The listing builds one solid part. Answer for the finished solid, in the listing's coordinates (mm). A direction names the side the tool comes from. Give positions to 0.01 mm unless a question says otherwise; leave off trailing zeros. Write each question's results on one line, items separated by ' | '. Start each with the question number.
from build123d import *

# Parameters (mm, degrees)
SKETCH1_W           = 38.1
SKETCH1_H           = 19.05
SKETCH1_W_2         = 31.75
SKETCH1_H_2         = 12.7
BOSS_EXTRUDE1_DEPTH = 304.8
SKETCH2_R           = 14.2875
CUT_EXTRUDE1_DEPTH  = 20.05
SKETCH3_R           = 3.175
CUT_EXTRUDE2_DEPTH  = 20.05
CUT_EXTRUDE3_DEPTH  = 20.05
CUT_EXTRUDE6_DEPTH  = 39.1
CUT_EXTRUDE7_REACH  = 21.05
CUT_EXTRUDE8_REACH  = 21.05
SKETCH9_R           = 6.35
CUT_EXTRUDE9_REACH  = 21.05
SKETCH10_R          = 2.667
SKETCH11_R          = 6.35
CUT_EXTRUDE10_DEPTH = 20.05
CUT_EXTRUDE11_DEPTH = 20.05


with BuildPart() as part:
    # Sketch1 → Boss-Extrude1 (new body)
    with BuildSketch(Plane.XY):
        with Locations((19.05, 9.525)):
            Rectangle(SKETCH1_W, SKETCH1_H)
        with Locations((19.05, 9.525)):
            Rectangle(SKETCH1_W_2, SKETCH1_H_2, mode=Mode.SUBTRACT)
    extrude(amount=BOSS_EXTRUDE1_DEPTH)

    # Sketch2 → Cut-Extrude1 (cut, through all)
    with BuildSketch(Plane(origin=(0, 19.05, 0), x_dir=(1, 0, 0), z_dir=(0, 1, 0))):
        with Locations((19.05, -19.05)):
            Circle(SKETCH2_R)
        with Locations((19.05, -222.25)):
            Circle(SKETCH2_R)
    extrude(amount=-CUT_EXTRUDE1_DEPTH, mode=Mode.SUBTRACT)

    # Sketch3 → Cut-Extrude2 (cut, through all)
    with BuildSketch(Plane(origin=(0, 19.05, 0), x_dir=(1, 0, 0), z_dir=(0, 1, 0))):
        with Locations((19.05, -295.275)):
            Circle(SKETCH3_R)
    extrude(amount=-CUT_EXTRUDE2_DEPTH, mode=Mode.SUBTRACT)

    # Sketch4 → Cut-Extrude3 (cut, through all)
    with BuildSketch(Plane(origin=(0, 19.05, 0), x_dir=(1, 0, 0), z_dir=(0, 1, 0))):
        with BuildLine():
            Line((31.75, -304.8), (31.75, -247.65))
            ThreePointArc((31.75, -247.65), (33.609871939, -243.159871939), (38.1, -241.3))
            Line((38.1, -241.3), (38.1, -304.8))
            Line((38.1, -304.8), (31.75, -304.8))
        make_face()
    extrude(amount=-CUT_EXTRUDE3_DEPTH, mode=Mode.SUBTRACT)

    # Sketch7 → Cut-Extrude6 (cut, through all)
    with BuildSketch(Plane.ZY):
        with BuildLine():
            Line((19.05, 14.2875), (57.15, 14.2875))
            ThreePointArc((57.15, 14.2875), (61.9125, 9.525), (57.15, 4.7625))
            Line((57.15, 4.7625), (19.05, 4.7625))
            ThreePointArc((19.05, 4.7625), (14.2875, 9.525), (19.05, 14.2875))
        make_face()
        with BuildLine():
            Line((76.2, 14.2875), (114.3, 14.2875))
            ThreePointArc((114.3, 14.2875), (119.0625, 9.525), (114.3, 4.7625))
            Line((114.3, 4.7625), (76.2, 4.7625))
            ThreePointArc((76.2, 4.7625), (71.4375, 9.525), (76.2, 14.2875))
        make_face()
        with BuildLine():
            Line((133.35, 14.2875), (171.45, 14.2875))
            ThreePointArc((171.45, 14.2875), (176.2125, 9.525), (171.45, 4.7625))
            Line((171.45, 4.7625), (133.35, 4.7625))
            ThreePointArc((133.35, 4.7625), (128.5875, 9.525), (133.35, 14.2875))
        make_face()
        with BuildLine():
            Line((190.5, 14.2875), (228.6, 14.2875))
            ThreePointArc((228.6, 14.2875), (233.3625, 9.525), (228.6, 4.7625))
            Line((228.6, 4.7625), (190.5, 4.7625))
            ThreePointArc((190.5, 4.7625), (185.7375, 9.525), (190.5, 14.2875))
        make_face()
        with BuildLine():
            Line((247.65, 14.2875), (285.75, 14.2875))
            ThreePointArc((285.75, 14.2875), (290.5125, 9.525), (285.75, 4.7625))
            Line((285.75, 4.7625), (247.65, 4.7625))
            ThreePointArc((247.65, 4.7625), (242.8875, 9.525), (247.65, 14.2875))
        make_face()
    extrude(amount=-CUT_EXTRUDE6_DEPTH, mode=Mode.SUBTRACT)

    # Sketch8 → Cut-Extrude7 (cut, up to next)
    with BuildSketch(Plane(origin=(0, 19.05, 0), x_dir=(1, 0, 0), z_dir=(0, 1, 0)), mode=Mode.PRIVATE) as cut_extrude7_sk1:
        with BuildLine():
            Line((11.1125, -44.45), (26.9875, -44.45))
            ThreePointArc((26.9875, -44.45), (31.477628061, -46.309871939), (33.3375, -50.8))
            Line((33.3375, -50.8), (33.3375, -190.5))
            ThreePointArc((33.3375, -190.5), (31.477628061, -194.990128061), (26.9875, -196.85))
            Line((26.9875, -196.85), (11.1125, -196.85))
            ThreePointArc((11.1125, -196.85), (6.622371939, -194.990128061), (4.7625, -190.5))
            Line((4.7625, -190.5), (4.7625, -50.8))
            ThreePointArc((4.7625, -50.8), (6.622371939, -46.309871939), (11.1125, -44.45))
        make_face()
    cut_extrude7_tool1 = extrude(cut_extrude7_sk1.sketch, amount=-CUT_EXTRUDE7_REACH, mode=Mode.PRIVATE) & part.part
    add(cut_extrude7_tool1.solids().sort_by_distance((19.05, 19.05, 120.65))[0], mode=Mode.SUBTRACT)

    # Sketch9 → Cut-Extrude8 (cut, up to next)
    with BuildSketch(Plane.XZ, mode=Mode.PRIVATE) as cut_extrude8_sk1:
        with Locations((9.525, 48.475738686)):
            Circle(SKETCH9_R)
    cut_extrude8_tool1 = extrude(cut_extrude8_sk1.sketch, amount=-CUT_EXTRUDE8_REACH, mode=Mode.PRIVATE) & part.part
    add(cut_extrude8_tool1.solids().sort_by_distance((9.525, 0, 48.475739))[0], mode=Mode.SUBTRACT)
    # Sketch9 → Cut-Extrude8 (cut, up to next)
    with BuildSketch(Plane.XZ, mode=Mode.PRIVATE) as cut_extrude8_sk2:
        with Locations((28.575, 59.474261314)):
            Circle(SKETCH9_R)
    cut_extrude8_tool2 = extrude(cut_extrude8_sk2.sketch, amount=-CUT_EXTRUDE8_REACH, mode=Mode.PRIVATE) & part.part
    add(cut_extrude8_tool2.solids().sort_by_distance((28.575, 0, 59.474261))[0], mode=Mode.SUBTRACT)
    # Sketch9 → Cut-Extrude8 (cut, up to next)
    with BuildSketch(Plane.XZ, mode=Mode.PRIVATE) as cut_extrude8_sk3:
        with Locations((9.525, 67.525738686)):
            Circle(SKETCH9_R)
    cut_extrude8_tool3 = extrude(cut_extrude8_sk3.sketch, amount=-CUT_EXTRUDE8_REACH, mode=Mode.PRIVATE) & part.part
    add(cut_extrude8_tool3.solids().sort_by_distance((9.525, 0, 67.525739))[0], mode=Mode.SUBTRACT)
    # Sketch9 → Cut-Extrude8 (cut, up to next)
    with BuildSketch(Plane.XZ, mode=Mode.PRIVATE) as cut_extrude8_sk4:
        with Locations((28.575, 78.524261314)):
            Circle(SKETCH9_R)
    cut_extrude8_tool4 = extrude(cut_extrude8_sk4.sketch, amount=-CUT_EXTRUDE8_REACH, mode=Mode.PRIVATE) & part.part
    add(cut_extrude8_tool4.solids().sort_by_distance((28.575, 0, 78.524261))[0], mode=Mode.SUBTRACT)
    # Sketch9 → Cut-Extrude8 (cut, up to next)
    with BuildSketch(Plane.XZ, mode=Mode.PRIVATE) as cut_extrude8_sk5:
        with Locations((9.525, 86.575738686)):
            Circle(SKETCH9_R)
    cut_extrude8_tool5 = extrude(cut_extrude8_sk5.sketch, amount=-CUT_EXTRUDE8_REACH, mode=Mode.PRIVATE) & part.part
    add(cut_extrude8_tool5.solids().sort_by_distance((9.525, 0, 86.575739))[0], mode=Mode.SUBTRACT)
    # Sketch9 → Cut-Extrude8 (cut, up to next)
    with BuildSketch(Plane.XZ, mode=Mode.PRIVATE) as cut_extrude8_sk6:
        with Locations((28.575, 97.574261314)):
            Circle(SKETCH9_R)
    cut_extrude8_tool6 = extrude(cut_extrude8_sk6.sketch, amount=-CUT_EXTRUDE8_REACH, mode=Mode.PRIVATE) & part.part
    add(cut_extrude8_tool6.solids().sort_by_distance((28.575, 0, 97.574261))[0], mode=Mode.SUBTRACT)
    # Sketch9 → Cut-Extrude8 (cut, up to next)
    with BuildSketch(Plane.XZ, mode=Mode.PRIVATE) as cut_extrude8_sk7:
        with Locations((9.525, 105.625738686)):
            Circle(SKETCH9_R)
    cut_extrude8_tool7 = extrude(cut_extrude8_sk7.sketch, amount=-CUT_EXTRUDE8_REACH, mode=Mode.PRIVATE) & part.part
    add(cut_extrude8_tool7.solids().sort_by_distance((9.525, 0, 105.625739))[0], mode=Mode.SUBTRACT)
    # Sketch9 → Cut-Extrude8 (cut, up to next)
    with BuildSketch(Plane.XZ, mode=Mode.PRIVATE) as cut_extrude8_sk8:
        with Locations((28.575, 116.624261314)):
            Circle(SKETCH9_R)
    cut_extrude8_tool8 = extrude(cut_extrude8_sk8.sketch, amount=-CUT_EXTRUDE8_REACH, mode=Mode.PRIVATE) & part.part
    add(cut_extrude8_tool8.solids().sort_by_distance((28.575, 0, 116.624261))[0], mode=Mode.SUBTRACT)
    # Sketch9 → Cut-Extrude8 (cut, up to next)
    with BuildSketch(Plane.XZ, mode=Mode.PRIVATE) as cut_extrude8_sk9:
        with Locations((9.525, 124.675738686)):
            Circle(SKETCH9_R)
    cut_extrude8_tool9 = extrude(cut_extrude8_sk9.sketch, amount=-CUT_EXTRUDE8_REACH, mode=Mode.PRIVATE) & part.part
    add(cut_extrude8_tool9.solids().sort_by_distance((9.525, 0, 124.675739))[0], mode=Mode.SUBTRACT)
    # Sketch9 → Cut-Extrude8 (cut, up to next)
    with BuildSketch(Plane.XZ, mode=Mode.PRIVATE) as cut_extrude8_sk10:
        with Locations((28.575, 135.674261314)):
            Circle(SKETCH9_R)
    cut_extrude8_tool10 = extrude(cut_extrude8_sk10.sketch, amount=-CUT_EXTRUDE8_REACH, mode=Mode.PRIVATE) & part.part
    add(cut_extrude8_tool10.solids().sort_by_distance((28.575, 0, 135.674261))[0], mode=Mode.SUBTRACT)
    # Sketch9 → Cut-Extrude8 (cut, up to next)
    with BuildSketch(Plane.XZ, mode=Mode.PRIVATE) as cut_extrude8_sk11:
        with Locations((9.525, 143.725738686)):
            Circle(SKETCH9_R)
    cut_extrude8_tool11 = extrude(cut_extrude8_sk11.sketch, amount=-CUT_EXTRUDE8_REACH, mode=Mode.PRIVATE) & part.part
    add(cut_extrude8_tool11.solids().sort_by_distance((9.525, 0, 143.725739))[0], mode=Mode.SUBTRACT)
    # Sketch9 → Cut-Extrude8 (cut, up to next)
    with BuildSketch(Plane.XZ, mode=Mode.PRIVATE) as cut_extrude8_sk12:
        with Locations((28.575, 154.724261314)):
            Circle(SKETCH9_R)
    cut_extrude8_tool12 = extrude(cut_extrude8_sk12.sketch, amount=-CUT_EXTRUDE8_REACH, mode=Mode.PRIVATE) & part.part
    add(cut_extrude8_tool12.solids().sort_by_distance((28.575, 0, 154.724261))[0], mode=Mode.SUBTRACT)
    # Sketch9 → Cut-Extrude8 (cut, up to next)
    with BuildSketch(Plane.XZ, mode=Mode.PRIVATE) as cut_extrude8_sk13:
        with Locations((9.525, 162.775738686)):
            Circle(SKETCH9_R)
    cut_extrude8_tool13 = extrude(cut_extrude8_sk13.sketch, amount=-CUT_EXTRUDE8_REACH, mode=Mode.PRIVATE) & part.part
    add(cut_extrude8_tool13.solids().sort_by_distance((9.525, 0, 162.775739))[0], mode=Mode.SUBTRACT)
    # Sketch9 → Cut-Extrude8 (cut, up to next)
    with BuildSketch(Plane.XZ, mode=Mode.PRIVATE) as cut_extrude8_sk14:
        with Locations((28.575, 173.774261314)):
            Circle(SKETCH9_R)
    cut_extrude8_tool14 = extrude(cut_extrude8_sk14.sketch, amount=-CUT_EXTRUDE8_REACH, mode=Mode.PRIVATE) & part.part
    add(cut_extrude8_tool14.solids().sort_by_distance((28.575, 0, 173.774261))[0], mode=Mode.SUBTRACT)
    # Sketch9 → Cut-Extrude8 (cut, up to next)
    with BuildSketch(Plane.XZ, mode=Mode.PRIVATE) as cut_extrude8_sk15:
        with Locations((9.525, 181.825738686)):
            Circle(SKETCH9_R)
    cut_extrude8_tool15 = extrude(cut_extrude8_sk15.sketch, amount=-CUT_EXTRUDE8_REACH, mode=Mode.PRIVATE) & part.part
    add(cut_extrude8_tool15.solids().sort_by_distance((9.525, 0, 181.825739))[0], mode=Mode.SUBTRACT)
    # Sketch9 → Cut-Extrude8 (cut, up to next)
    with BuildSketch(Plane.XZ, mode=Mode.PRIVATE) as cut_extrude8_sk16:
        with Locations((28.575, 192.824261314)):
            Circle(SKETCH9_R)
    cut_extrude8_tool16 = extrude(cut_extrude8_sk16.sketch, amount=-CUT_EXTRUDE8_REACH, mode=Mode.PRIVATE) & part.part
    add(cut_extrude8_tool16.solids().sort_by_distance((28.575, 0, 192.824261))[0], mode=Mode.SUBTRACT)

    # Sketch10 → Cut-Extrude9 (cut, up to next)
    with BuildSketch(Plane.XZ, mode=Mode.PRIVATE) as cut_extrude9_sk1:
        with Locations((19.05, 130.175)):
            Circle(SKETCH10_R)
    cut_extrude9_tool1 = extrude(cut_extrude9_sk1.sketch, amount=-CUT_EXTRUDE9_REACH, mode=Mode.PRIVATE) & part.part
    add(cut_extrude9_tool1.solids().sort_by_distance((19.05, 0, 130.175))[0], mode=Mode.SUBTRACT)

    # Sketch11 → Cut-Extrude10 (cut, through all)
    with BuildSketch(Plane(origin=(0, 19.05, 0), x_dir=(1, 0, 0), z_dir=(0, 1, 0))):
        with Locations((12.7, -245.927225036)):
            Circle(SKETCH11_R)
        with Locations((12.7, -264.977225036)):
            Circle(SKETCH11_R)
        with Locations((12.7, -284.027225036)):
            Circle(SKETCH11_R)
    extrude(amount=-CUT_EXTRUDE10_DEPTH, mode=Mode.SUBTRACT)

    # Sketch12 → Cut-Extrude11 (cut, through all)
    with BuildSketch(Plane(origin=(0, 19.05, 0), x_dir=(1, 0, 0), z_dir=(0, 1, 0))):
        Polygon((28.575, 0), (38.1, -9.525), (38.1, 0), align=None)
        Polygon((0, 0), (9.525, 0), (0, -9.525), align=None)
        Polygon((9.525, -304.8), (0, -295.275), (0, -304.8), align=None)
        Polygon((31.75, -304.8), (22.225, -304.8), (31.75, -295.275), align=None)
    extrude(amount=-CUT_EXTRUDE11_DEPTH, mode=Mode.SUBTRACT)


solid = part.part
1. Consider probe 1 along X at (y, z) = (6.5, 180) (3 decimals); probe 2 along Y at (x, z) = (29, 205) (3 decimals); probe 3 along Z at (x, y) = (30.5, 16.25) (3 decimals). Determine where each line is inside the solid, lowest interval first. Write a range as [from, to].
2. Each of these flat-tipped pins is pushed along its axis until it touches: pin 1 Ø10 at (x, z) = (9.52, 105.63) entering from -Y (3 decimals); pin 2 Ø1 at (x, y) = (24, 5) entering from +Z. Where does it stop, or does it pass through?
3. A tool of negligible diameter and unlimited length cuts with its end or side. For faces 1 (the cylindrical face through (22.23, 1.57, 193.1)), 2 (the flat face through (19, 3.175, 150)), 3 (the cylindrical face through (17.084, 1.565, 131.977)), 4 (the cylindrical face through (1.57, 9.63, 61.91)), from which of +Z, -Z, +X, -X, +Y, -Y can it reach the whole face along a straight path? Write none if from no direction.
4. The mould has two halves that part along Z. Classify faces 5 (the cylindrical face through (23.536, 1.565, 93.71)), 6 (the flat face through (2, 19.05, 186)), 7 (the flat face through (2.713, 9.658, 297.988)): pulls with the +Z half, pulls with the -Z half, needs draft (parallel to the pull), parting line crosses it, or undercut.
5. Section A-A (z = 222.25) is taken. Give the number of separate pieces and of enclosed holes in the cut face, then the cut area to 3 significant figures.
Results:
1) probe 1: x = [0, 3.175], [34.925, 38.1] | probe 2: y = [0, 3.175], [15.875, 19.05] | probe 3: z = [1.925, 10.504], [27.596, 45.51], [195.79, 213.704], [230.796, 296.525]
2) pin 1: stops at y = 15.875 | pin 2: passes through
3) face 1: -Y | face 2: +Z, -Z | face 3: +Y, -Y | face 4: +X, -X
4) face 5: undercut | face 6: needs draft | face 7: pulls with the +Z half
5) separate pieces: 4 | enclosed holes: 0 | area: 80.6 mm²
